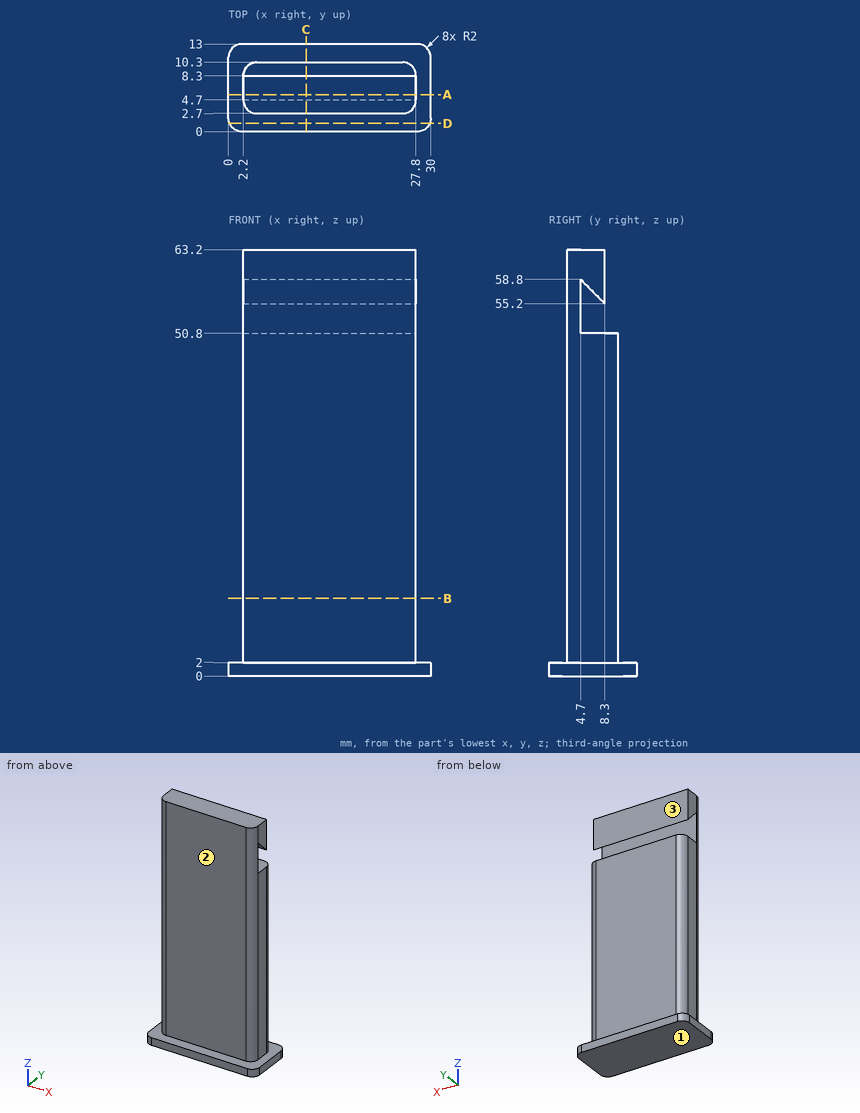
Part print with two shaded views. Sizes in mm from the minimum x, y, z corner. A direction names the side the tool comes from. Coordinates: 2 decimals unless noted, no trailing zeros. Write each loop counter-clockwise with the first axis right and the second up, starting at its lowest first coordinate (ties: lowest second). Pieces come first, ordered by that corner, then holes. Notation, with made-up numbers: (0, 87) -> (5, 87) arc R24 ccw to (5, 97) -> close; hole circle Ø3 at (-10, -38.75). An arc over 180 degrees is marked (long way). Return JSON: item names as keys, results as strings. Group by question number.
Q1. Which spindle directions (+Z, -Z, +X, -X, +Y, -Y) get a long thin tool onto all of the face, cutting with end or side? Do the marked faces 1, 2 and 3. Say none if no direction does.
Q2. Flat gauge pins, fed straight in: pin 1 (8 mm diameter, centred on x = 6, z = 53.5, fed in from +Y); pin 2 (4 mm diameter, centred on y = 10, z = 31, fed in from +X); pin 3 (1.1 mm diameter, centred on y = 7, z = 57.5, fed in from -X). Where does each tip first touch, or does it go through?
Q3. Cut at A-A, the plane y = 5.5. Give the cut face in (x, z), then the cut area to 3 significant figures.
Q4. Cut at C-C, the plane x = 11.5. Give the cut face in (y, z), then the cut area to 3 significant figures.
Q5. Cut at B-B, the plane z = 11.5. Give the cut face in (x, y), then the cut area to 3 significant figures.
Q6. Cut at D-D, the plane y = 1.25. Give the cut face in (x, z).
Q7. Drill centre lines: line 1 (Z direction, x = 11.25, y = 9); line 2 (Y direction, x = 20.75, z = 12); line 3 (X direction, y = 4.5, z = 30.5). Where is each one in solid material? Low to high.
Returned:
{
 "1": {"face 1": "-Z, +X, -X, +Y, -Y", "face 2": "+Z, +X, -X, -Y", "face 3": "+Z, +X, -X, +Y"},
 "2": {"pin 1": "stops at y = 10.3", "pin 2": "stops at x = 27.8", "pin 3": "stops at x = 2.2"},
 "3": {"outline": "(0, 0) -> (30, 0) -> (30, 2) -> (27.8, 2) -> (27.8, 50.8) -> (2.2, 50.8) -> (2.2, 2) -> (0, 2) -> close; (2.2, 58) -> (27.8, 58) -> (27.8, 63.2) -> (2.2, 63.2) -> close", "area": "1,440 mm2"},
 "4": {"outline": "(0, 0) -> (13, 0) -> (13, 2) -> (10.3, 2) -> (10.3, 50.8) -> (4.7, 50.8) -> (4.7, 58.8) -> (8.3, 55.2) -> (8.3, 63.2) -> (2.7, 63.2) -> (2.7, 2) -> (0, 2) -> close", "area": "444 mm2"},
 "5": {"outline": "(2.2, 4.7) arc R2 ccw to (4.2, 2.7) -> (25.8, 2.7) arc R2 ccw to (27.8, 4.7) -> (27.8, 8.3) arc R2 ccw to (25.8, 10.3) -> (4.2, 10.3) arc R2 ccw to (2.2, 8.3) -> close", "area": "191 mm2"},
 "6": {"outline": "(0.15, 0) -> (29.85, 0) -> (29.85, 2) -> (0.15, 2) -> close"},
 "7": {"line 1": "z = 0 to 50.8", "line 2": "y = 2.7 to 10.3", "line 3": "x = 2.21 to 27.79"}
}
